Check sheet for the modelled part. Datum: model origin and axes. Units: mm. A direction names the side the tool comes from. Round coordinates to 2 decimals unless told otherwise and drop trailing zeros. Loops run counter-clockwise (first coordinate to the right, second up) from the corner with the lowest first, then second, coordinate; pieces in that order, holes last. Notation, with made-up numbers: M 63,1 L 118,1 A10 ccw 118,20 Z; hole C 57.25,-35 d1. An arc over 180 degrees is marked long. One line per question, with ' | ' between items. Start each with the question number.
(1) Tool access check on faces 1 (the face through (-77.15, 5.07, 96.99)), 2 (the face through (0.601, 9.014, -93.092)). Record the directions out of +Z, -Z, +X, -X, +Y, -Y that give a thin tool (end or side, any length) a straight path to the whole face; none if there is none.
(2) Go/stop test with a flat-tipped pin: P1, Ø1.2, axis at x = -0.5, z = -94.5, coming from the +Y side. Record where the tip stops, or that it passes through.
(3) Draft check along X on faces 3 (the face through (0, 8, -95)), 4 (the face through (-1, 0, -1)), 5 (the face through (76.99, 5.07, 97.15)). Enter one of: +X half, -X half, draft (parallel to the pull), parting line (faces both ways), or undercut.
(4) Thickness scan on probe 1 along Z at (x, y) = (52, 9); probe 2 along X at (y, z) = (8.25, 68); probe 3 along Y at (x, z) = (29, 36). Record the ranges inside material, lowest first. Write a range as [from, to].
(5) Section check A-A (x = 29). Record the boundary of the cut face in (y, z), and give its area (3 significant figures).
(6) Section check B-B (z = -67). Record the boundary of the cut face in (x, y).
```python
from build123d import *

# Parameters (mm, degrees)
SKETCH_1_W          = 160
SKETCH_1_H          = 200
EXTRUDE_1_DEPTH     = 10
SKETCH_2_R          = 2
SKETCH_2_W          = 140
SKETCH_2_H          = 180
CUT_EXTRUDE_1_DEPTH = 2
FILLET_1_R          = 10
FILLET_2_R          = 2


with BuildPart() as part:
    # 草图1 → 凸台-拉伸1 (new body)
    with BuildSketch(Plane(origin=(0, 0, 0), x_dir=(1, 0, 0), z_dir=(0, 1, 0))):
        Rectangle(SKETCH_1_W, SKETCH_1_H)
    extrude(amount=EXTRUDE_1_DEPTH)

    # 草图2 → 切除-拉伸1 (cut)
    with BuildSketch(Plane(origin=(0, 10, 0), x_dir=(1, 0, 0), z_dir=(0, 1, 0))):
        with Locations(Location((0, 95, 0), (0, 0, 270))):
            Circle(SKETCH_2_R)
        Rectangle(SKETCH_2_W, SKETCH_2_H)
    extrude(amount=-CUT_EXTRUDE_1_DEPTH, mode=Mode.SUBTRACT)

    # 圆角1
    fillet_1_edges = [part.edges().sort_by_distance(p)[0] for p in [
        (-80, 5, -100),
        (80, 5, -100),
        (80, 5, 100),
        (-80, 5, 100),
    ]]
    fillet(fillet_1_edges, radius=FILLET_1_R)

    # 圆角2
    fillet_2_edges = [part.edges().sort_by_distance(p)[0] for p in [
        (-70, 9, 90),
        (-70, 9, -90),
        (70, 9, -90),
        (70, 9, 90),
    ]]
    fillet(fillet_2_edges, radius=FILLET_2_R)


solid = part.part
```
The answers:
1) face 1: +Z, -X, +Y, -Y | face 2: +Y
2) P1: y = 8
3) face 3: undercut | face 4: draft | face 5: +X half
4) probe 1: [-100, -90], [90, 100] | probe 2: [-80, -70], [70, 80] | probe 3: [0, 8]
5) outline: M 0,-100 L 10,-100 L 10,-90 L 8,-90 L 8,90 L 10,90 L 10,100 L 0,100 Z | area: 1,640 mm²
6) outline: M -80,0 L 80,0 L 80,10 L 70,10 L 70,8 L -70,8 L -70,10 L -80,10 Z
